from build123d import *

# Parameters (mm, degrees)
SKETCH1_W          = 25.4
SKETCH1_H          = 177.8
BASE_EXTRUDE_DEPTH = 22.86
SKETCH2_R          = 7.62
CUT_EXTRUDE1_DEPTH = 78.74
FILLET1_R          = 7.62


with BuildPart() as part:
    # Sketch1 → Base-Extrude (new body)
    with BuildSketch(Plane.XY):
        with Locations((-7.849662618, -19.144264507)):
            Rectangle(SKETCH1_W, SKETCH1_H)
    extrude(amount=BASE_EXTRUDE_DEPTH)

    # Sketch2 → Cut-Extrude1 (cut)
    with BuildSketch(Plane.XY.offset(22.86)):
        with Locations((-7.849662618, -95.344264507)):
            Circle(SKETCH2_R)
        with Locations((-7.849662618, 57.055735493)):
            Circle(SKETCH2_R)
    extrude(amount=-CUT_EXTRUDE1_DEPTH, mode=Mode.SUBTRACT)

    # Fillet1
    fillet1_edges = [part.edges().sort_by_distance(p)[0] for p in [
        (-20.549662618, 69.755735493, 11.43),
        (4.850337382, 69.755735493, 11.43),
        (4.850337382, -108.044264507, 11.43),
        (-20.549662618, -108.044264507, 11.43),
    ]]
    fillet(fillet1_edges, radius=FILLET1_R)


solid = part.part
Here's how the part is built. I have some questions about the finished solid (model axes, mm). Give positions to 0.01 mm unless a question says otherwise; leave off trailing zeros. Order: outer loops, then holes, each group sorted by start corner. A loop starts at its lowest first (then second) coordinate and runs counter-clockwise, first axis right, second up. Notation, with made-up numbers: M 78.25,-12 L 133.25,-12 A8 cw 133.25,-3 Z; hole C -3,25.5 d8. An arc over 180 degrees is marked long. Answer as a JSON object with one key per item and string values. Group by question number.
1) We'd pull the mould along X, two halves only. Please class faces 1 (the cylindrical face through (-8.84, 64.61, 11.59)), 2 (the cylindrical face through (2.56, 67.58, 11.59)), 3 (the flat face through (-8, 69.756, 11)): pulls with the +X half, pulls with the -X half, needs draft (parallel to the pull), parting line crosses it, or undercut.
2) Suppose I cut it at B-B, the plane y = 53. Write out the boundary of the cut face in (x, z), plus the area to 3 significant figures.
3) Suppose I cut it at C-C, the plane z = 12.25. Write out the boundary of the cut face in (x, y), plus the area to 3 significant figures.
4) I'm going to push flat-ended pins straight in: pin 1 Ø1 at (x, z) = (-17.5, 4) entering from +Y; pin 2 Ø1 at (x, z) = (-14, 20) entering from +Y; pin 3 Ø12 at (x, y) = (-2, -79.5) entering from -Z; pin 4 Ø6 at (x, z) = (-17, 7.5) entering from -Y. Where does each tip first touch, or does it pass through?
5) Please list where these lines run through material, in increasing order: L1, parallel to Y at x = -4, z = 19.75; L2, parallel to Y at x = -9.75, z = 15.75; L3, parallel to Y at x = -17.5, z = 21.75. Write a range as [from, to].
6) Suppose I cut it at A-A, the plane x = -10.25. Write out the boundary of the cut face in (y, z).
Results found:
{
 "1": {"face 1": "undercut", "face 2": "pulls with the +X half", "face 3": "needs draft"},
 "2": {"outline": "M -20.55,0 L -14.3,0 L -14.3,22.86 L -20.55,22.86 Z; M -1.4,0 L 4.85,0 L 4.85,22.86 L -1.4,22.86 Z", "area": "286 mm²"},
 "3": {"outline": "M -20.55,-100.42 A7.62 ccw -12.93,-108.04 L -2.77,-108.04 A7.62 ccw 4.85,-100.42 L 4.85,62.14 A7.62 ccw -2.77,69.76 L -12.93,69.76 A7.62 ccw -20.55,62.14 Z; hole C -7.85,-95.34 d15.24; hole C -7.85,57.06 d15.24", "area": "4,100 mm²"},
 "4": {"pin 1": "y = 68.58", "pin 2": "y = 69.73", "pin 3": "z = 0", "pin 4": "y = -107.97"},
 "5": {"L1": "[-108.04, -101.92], [-88.77, 50.48], [63.63, 69.76]", "L2": "[-108.04, -102.72], [-87.97, 49.68], [64.43, 69.76]", "L3": "[-106.52, 68.23]"},
 "6": {"outline": "M -108.04,0 L -102.58,0 L -102.58,22.86 L -108.04,22.86 Z; M -88.11,0 L 49.82,0 L 49.82,22.86 L -88.11,22.86 Z; M 64.29,0 L 69.76,0 L 69.76,22.86 L 64.29,22.86 Z"}
}
